Design review of the part shown in the three views and the two pictorial views. Dimensions are in mm from the part's minimum x, y and z. A direction names the side the tool comes from. Coordinates: 2 decimals unless noted, no trailing zeros. Order: outer loops, then holes, each group sorted by start corner. A loop starts at its lowest first (then second) coordinate and runs counter-clockwise, first axis right, second up. Notation, with made-up numbers: (54, -30.5) -> (90, -30.5) arc R23 cw to (90, 2.5) -> close; hole circle Ø10 at (58.5, -9.75). An arc over 180 degrees is marked (long way). Write item = value, one per line. Start each with the question number.
1) Machinability: for the marked faces 1 and 2, which of the approach directions +Z, -Z, +X, -X, +Y, -Y give a long, thin tool a straight path to every point of the face, cutting with its end or side? Answer none if there is none.
2) Wall thickness on probe 1 along Y at (x, z) = (4, 3.95); probe 2 along X at (y, z) = (5.25, 15.25); probe 3 along Z at (x, y) = (3.5, 4): over which ranges is each line inside the solid? List them lowest first. Write a range as [from, to].
3) Consider section C-C on z = 17.75. Give the boundary of the cut face in (x, y).
4) Insertion check: pin 1 Ø2.5 at (x, y) = (4, 4) entering from +Z. The pin has a flat end and moves straight along its axis. Give the tip position at first contact, or say it passes through.
5) Consider section D-D on z = 10. Give the boundary of the cut face in (x, y), and give its area (3 significant figures).
6) Consider section A-A on x = 4. Give the boundary of the cut face in (y, z).
7) Draft analysis for pull direction Y (two halves, no side actions). For the marked faces 3, 4 and 5, state which applies: +Y half, -Y half, draft (parallel to the pull), parting line (faces both ways), or undercut.
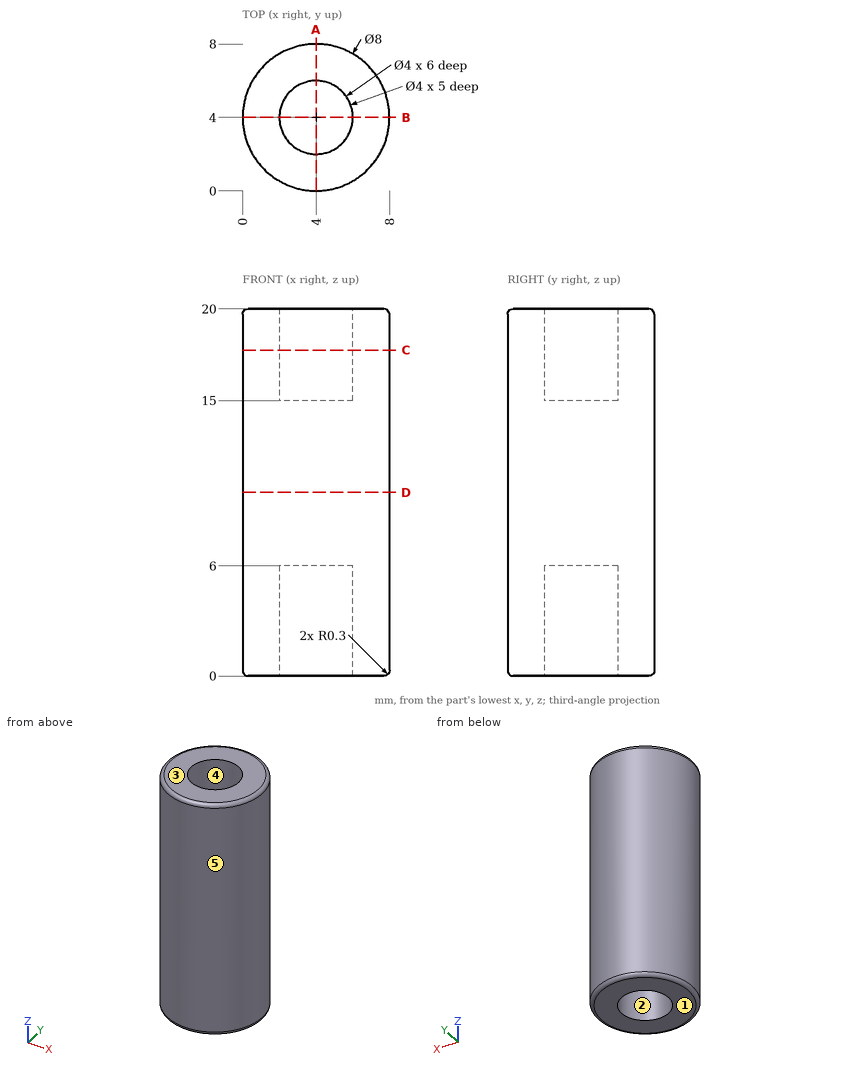
Answer sheet:
q1.face_1 = -Z, +X, -X, +Y, -Y
q1.face_2 = -Z
q2.probe_1 = [0, 2], [6, 8]
q2.probe_2 = [0.2, 2.44], [5.56, 7.8]
q2.probe_3 = [6, 15]
q3.outline = circle Ø8 at (4, 4); hole circle Ø4 at (4, 4)
q4.pin_1 = 15
q5.outline = circle Ø8 at (4, 4)
q5.area = 50.3 mm2
q6.outline = (0, 0.3) arc R0.3 ccw to (0.3, 0) -> (2, 0) -> (2, 6) -> (6, 6) -> (6, 0) -> (7.7, 0) arc R0.3 ccw to (8, 0.3) -> (8, 19.7) arc R0.3 ccw to (7.7, 20) -> (6, 20) -> (6, 15) -> (2, 15) -> (2, 20) -> (0.3, 20) arc R0.3 ccw to (0, 19.7) -> close
q7.face_3 = draft
q7.face_4 = undercut
q7.face_5 = parting line
